from build123d import *

# Parameters (mm, degrees)
F0_W     = 1190
F0_H     = 920
F1_DEPTH = 8
F2_W     = 50
F2_H     = 920
F3_DEPTH = 80


with BuildPart() as f1:
    # F0 (on Front) → F1 (new body)
    with BuildSketch(Plane.XZ):
        with Locations((595, 460)):
            Rectangle(F0_W, F0_H)
    extrude(amount=F1_DEPTH)

    # F2 (on face) → F3 (join)
    with BuildSketch(Plane(origin=(0, 0, 0), x_dir=(-1, 0, 0), z_dir=(0, 1, 0))):
        with Locations((-892.5, 460)):
            Rectangle(F2_W, F2_H)
        with Locations((-297.5, 460)):
            Rectangle(F2_W, F2_H)
    extrude(amount=F3_DEPTH)


solid = f1.part
For this review, take the finished solid that the model builds, in its own axes (mm). A direction names the side the tool comes from. Give positions to 0.01 mm unless a question says otherwise; leave off trailing zeros. Loops run counter-clockwise (first coordinate to the right, second up) from the corner with the lowest first, then second, coordinate; pieces in that order, holes last. Notation, with made-up numbers: M 6.5,75 L 45.5,75 A25 cw 45.5,106 Z; hole C 7.25,-15 d8. An arc over 180 degrees is marked long. Answer as a JSON object with one key per item and string values. Group by question number.
Q1. Add section A-A on y = 44. Give the boundary of the cut face in (x, z), and give its area (3 significant figures).
Q2. For probe 1 along X at (y, z) = (10.5, 273); probe 2 along Y at (x, z) = (532, 232.5), list the stretches that pass through material, from the lowest coordinate up. Write a range as [from, to].
Q3. Add section B-B on z = 554.5. Give the boundary of the cut face in (x, y).
Q4. Insertion check: P1, Ø1.5, axis at y = 10.5, z = 785, coming from the +X side; P2, Ø8, axis at x = 211.5, z = 336.5, coming from the +Y side. Each pin has a flat end and moves straight along its axis. Give the tip position at first contact, or say it passes through.
Q5. Add section C-C on x = 481.5. Give the boundary of the cut face in (y, z), and give its area (3 significant figures).
Q6. Tool access review of faces 1 (the flat face through (298, 80, 466)), 2 (the flat face through (1052, 0, 466)), 3 (the flat face through (322.5, 39, 454)): name each direction out of +Z, -Z, +X, -X, +Y, -Y from which nothing blocks a thin tool from reaching the whole face with its end or side.
Q7. Mouldability with a two-part tool opening along X and no side actions: class faces 4 (the flat face through (272.5, 39, 454)), 5 (the flat face through (591, 0, 466)), 6 (the flat face through (134, 0, 466)) as +X half, -X half, draft (parallel to the pull), parting line (faces both ways), or undercut.
Checked values:
{
 "1": {"outline": "M 272.5,0 L 322.5,0 L 322.5,920 L 272.5,920 Z; M 867.5,0 L 917.5,0 L 917.5,920 L 867.5,920 Z", "area": "92,000 mm²"},
 "2": {"probe 1": "[272.5, 322.5], [867.5, 917.5]", "probe 2": "[-8, 0]"},
 "3": {"outline": "M 0,-8 L 1190,-8 L 1190,0 L 917.5,0 L 917.5,80 L 867.5,80 L 867.5,0 L 322.5,0 L 322.5,80 L 272.5,80 L 272.5,0 L 0,0 Z"},
 "4": {"P1": "x = 917.5", "P2": "y = 0"},
 "5": {"outline": "M -8,0 L 0,0 L 0,920 L -8,920 Z", "area": "7,360 mm²"},
 "6": {"face 1": "+Z, -Z, +X, -X, +Y", "face 2": "+Z, -Z, +X, +Y", "face 3": "+Z, -Z, +Y"},
 "7": {"face 4": "-X half", "face 5": "undercut", "face 6": "draft"}
}
